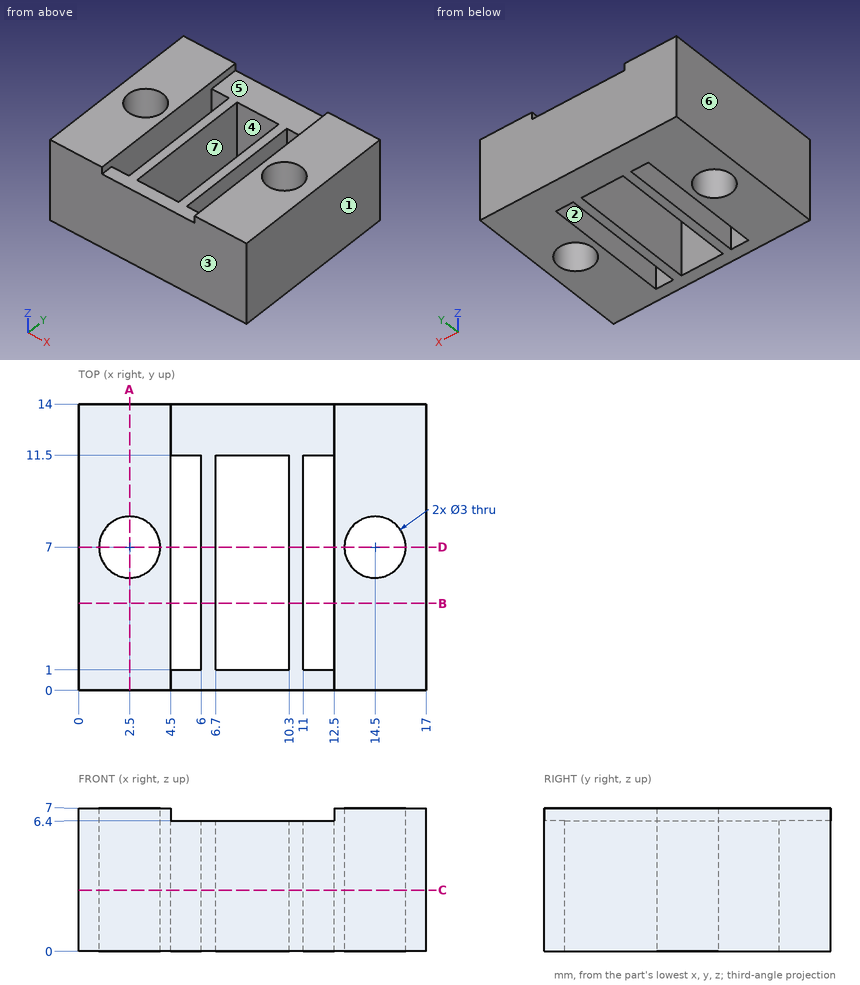
Design review of the part shown in the three views and the two pictorial views. Dimensions are in mm from the part's minimum x, y and z. A direction names the side the tool comes from. Coordinates: 2 decimals unless noted, no trailing zeros. Order: outer loops, then holes, each group sorted by start corner. A loop starts at its lowest first (then second) coordinate and runs counter-clockwise, first axis right, second up. Notation, with made-up numbers: (54.5, -4) - (86.5, -4) arc R24 ccw to (86.5, 34) - close; hole circle Ø2 at (34.25, 64). An arc over 180 degrees is marked (long way). Answer as CSV lines item,"result". Start each with the question number.
1) Machinability: for the marked faces 5, 6 and 7, which of the approach directions +Z, -Z, +X, -X, +Y, -Y give a long, thin tool a straight path to every point of the face, cutting with its end or side? Answer none if there is none.
2) Add section B-B (y = 4.25). State the section outline as (x, z) points.
3) Add section D-D (y = 7). State the section outline as (x, z) points.
4) Add section C-C (z = 3). State the section outline as (x, y) points.
5) Add section A-A (x = 2.5). State the section outline as (y, z) points, then the cut area to 3 significant figures.
6) Draft analysis for pull direction X (two halves, no side actions). For the marked faces 1, 2, 3 and 4, state which applies: +X half, -X half, draft (parallel to the pull), parting line (faces both ways), or undercut.
7) To check wall thickness, follow line 1 along X through (y, z) = (1.75, 2.5); line 2 along Y through (x, z) = (5.75, 2.75); line 3 along Y through (x, z) = (14.5, 3.75). State the ranges of each line that lie inside material, in increasing order. Write a range as [from, to].
Result:
1,face 5,"+Z, +Y, -Y"
1,face 6,"+Z, -Z, -X, +Y, -Y"
1,face 7,"+Z, -Z"
2,outline,"(0, 0) - (4.5, 0) - (4.5, 7) - (0, 7) - close; (6, 0) - (6.7, 0) - (6.7, 6.4) - (6, 6.4) - close; (10.3, 0) - (11, 0) - (11, 6.4) - (10.3, 6.4) - close; (12.5, 0) - (17, 0) - (17, 7) - (12.5, 7) - close"
3,outline,"(0, 0) - (1, 0) - (1, 7) - (0, 7) - close; (4, 0) - (4.5, 0) - (4.5, 7) - (4, 7) - close; (6, 0) - (6.7, 0) - (6.7, 6.4) - (6, 6.4) - close; (10.3, 0) - (11, 0) - (11, 6.4) - (10.3, 6.4) - close; (12.5, 0) - (13, 0) - (13, 7) - (12.5, 7) - close; (16, 0) - (17, 0) - (17, 7) - (16, 7) - close"
4,outline,"(0, 0) - (17, 0) - (17, 14) - (0, 14) - close; hole circle Ø3 at (2.5, 7); hole (4.5, 1) - (6, 1) - (6, 11.5) - (4.5, 11.5) - close; hole (6.7, 1) - (10.3, 1) - (10.3, 11.5) - (6.7, 11.5) - close; hole (11, 1) - (12.5, 1) - (12.5, 11.5) - (11, 11.5) - close; hole circle Ø3 at (14.5, 7)"
5,outline,"(0, 0) - (5.5, 0) - (5.5, 7) - (0, 7) - close; (8.5, 0) - (14, 0) - (14, 7) - (8.5, 7) - close"
5,area,"77.0 mm^2"
6,face 1,"+X half"
6,face 2,"undercut"
6,face 3,"draft"
6,face 4,"undercut"
7,line 1,"[0, 4.5], [6, 6.7], [10.3, 11], [12.5, 17]"
7,line 2,"[0, 1], [11.5, 14]"
7,line 3,"[0, 5.5], [8.5, 14]"
